Design review of the part built by this model. Coordinates are the model's own, in mm. A direction names the side the tool comes from. Coordinates: 2 decimals unless noted, no trailing zeros. Loops run counter-clockwise (first coordinate to the right, second up) from the corner with the lowest first, then second, coordinate; pieces in that order, holes last. Notation, with made-up numbers: M 11,63 L 40,63 A23 cw 40,92 Z; hole C 56,-31.75 d10. An arc over 180 degrees is marked long. Answer as CSV lines item,"result". Start each with the question number.
from build123d import *

# Parameters (mm, degrees)
EXTRUDE_1_DEPTH     = 350
OTHER_START         = -25
OTHER_1_DEPTH       = 50
SKETCH_4_R          = 4.1
CUT_EXTRUDE_1_DEPTH = 352.975510618


# Read off the part's stored shape, not the designer's step: Полость1
with BuildPart() as part:
    # Эскиз1 → Бобышка-Вытянуть1 (new body)
    with BuildSketch(Plane.XY):
        with BuildLine():
            Line((-4.4, -25), (-4.4, 25))
            Line((-4.4, 25), (27.6, 25))
            Line((27.6, 25), (27.6, 23.1))
            ThreePointArc((27.6, 23.1), (26.867766953, 21.332233047), (25.1, 20.6))
            Line((25.1, 20.6), (6, 20.6))
            ThreePointArc((6, 20.6), (1.757359313, 18.842640687), (0, 14.6))
            Line((0, 14.6), (0, -14.6))
            ThreePointArc((0, -14.6), (1.757359313, -18.842640687), (6, -20.6))
            Line((6, -20.6), (25.1, -20.6))
            ThreePointArc((25.1, -20.6), (26.867766953, -21.332233047), (27.6, -23.1))
            Line((27.6, -23.1), (27.6, -25))
            Line((27.6, -25), (-4.4, -25))
        make_face()
    extrude(amount=EXTRUDE_1_DEPTH)

    # Полость1 outline → Полость1 (cut)
    with BuildSketch(Plane(origin=(0, 0, 0), x_dir=(1, 0, 0), z_dir=(0, 1, 0)).offset(OTHER_START)):
        with BuildLine():
            ThreePointArc((3, -291), (0.878679656, -291.878679656), (0, -294))
            Line((0, -294), (0, -328))
            ThreePointArc((0, -328), (0.878679656, -330.121320344), (3, -331))
            Line((3, -331), (27.6, -331))
            Line((27.6, -331), (27.6, -291))
            Line((27.6, -291), (3, -291))
        make_face()
    extrude(amount=OTHER_1_DEPTH, mode=Mode.SUBTRACT)

    # Эскиз4 → Вырез-Вытянуть1 (cut, through all)
    with BuildSketch(Plane(origin=(0, 0, 0), x_dir=(0, 0, -1), z_dir=(1, 0, 0))):
        with Locations((-340.5, 0)):
            Circle(SKETCH_4_R)
        with Locations((-281.5, 0)):
            Circle(SKETCH_4_R)
    extrude(amount=-CUT_EXTRUDE_1_DEPTH, mode=Mode.SUBTRACT)

    # Зеркальное отражение1: part across plane


with BuildPart() as part_1:
    add(part.part)
    add(part.part.mirror(Plane(origin=(25.1, 23.1, 0), x_dir=(1, 0, 0), z_dir=(0, 0, -1))))


solid = part_1.part
Item 1: Add section B-B (z = 64.5). Give the boundary of the cut face in (x, y), plus the area to 3 significant figures.
Item 2: For pin 1 (6 mm diameter, centred on y = 16, z = -75.5, fed in from +X); pin 2 (5 mm diameter, centred on y = 15, z = -254, fed in from +X); pin 3 (2 mm diameter, centred on y = -1, z = 90, fed in from +X), all flat-tipped, find the tip position at first contact; note any pin that passes through.
Item 3: Add section A-A (x = 13). Give the boundary of the cut face in (y, z), plus the area to 3 significant figures.
Item 4: Mouldability with a two-part tool opening along Y and no side actions: class faces 1 (the face through (12, -25, 5)), 2 (the face through (0, 0, 5)), 3 (the face through (-0.2, 0.1, 350)), 4 (the face through (11, 25, 5)) as released by +Y, released by -Y, zero draft, split by the parting line, or undercut.
Item 5: For faces 5 (the face through (-4.4, 0, 5)), 6 (the face through (16, 20.6, 340)), list the 3-axis set-ups (+Z, -Z, +X, -X, +Y, -Y) from which the entire face can be reached by the end or side of a thin tool; tool diameter is ignored.
Item 6: For line 1 along Y through (x, z) = (8, 8); line 2 along Z through (x, y) = (21, -21.5); line 3 along Y through (x, z) = (-3.2, -281.5), list the stretches that pass through material, from the lowest coordinate up. Write a range as from..to.
Response:
1,outline,"M -4.4,-25 L 27.6,-25 L 27.6,-23.1 A2.5 ccw 25.1,-20.6 L 6,-20.6 A6 cw 0,-14.6 L 0,14.6 A6 cw 6,20.6 L 25.1,20.6 A2.5 ccw 27.6,23.1 L 27.6,25 L -4.4,25 Z"
1,area,"476 mm²"
2,pin 1,"x = 1.92"
2,pin 2,"x = 0.75"
2,pin 3,"x = 0"
3,outline,"M -25,-350 L -20.6,-350 L -20.6,-331 L -25,-331 Z; M -25,-291 L -20.6,-291 L -20.6,291 L -25,291 Z; M -25,331 L -20.6,331 L -20.6,350 L -25,350 Z; M 20.6,-350 L 25,-350 L 25,-331 L 20.6,-331 Z; M 20.6,-291 L 25,-291 L 25,291 L 20.6,291 Z; M 20.6,331 L 25,331 L 25,350 L 20.6,350 Z"
3,area,"5,460 mm²"
4,face 1,"released by -Y"
4,face 2,"undercut"
4,face 3,"zero draft"
4,face 4,"released by +Y"
5,face 5,"+Z, -Z, -X, +Y, -Y"
5,face 6,"+Z, -Z, +X"
6,line 1,"-25..-20.6, 20.6..25"
6,line 2,"-350..-331, -291..291, 331..350"
6,line 3,"-25..-4.1, 4.1..25"
